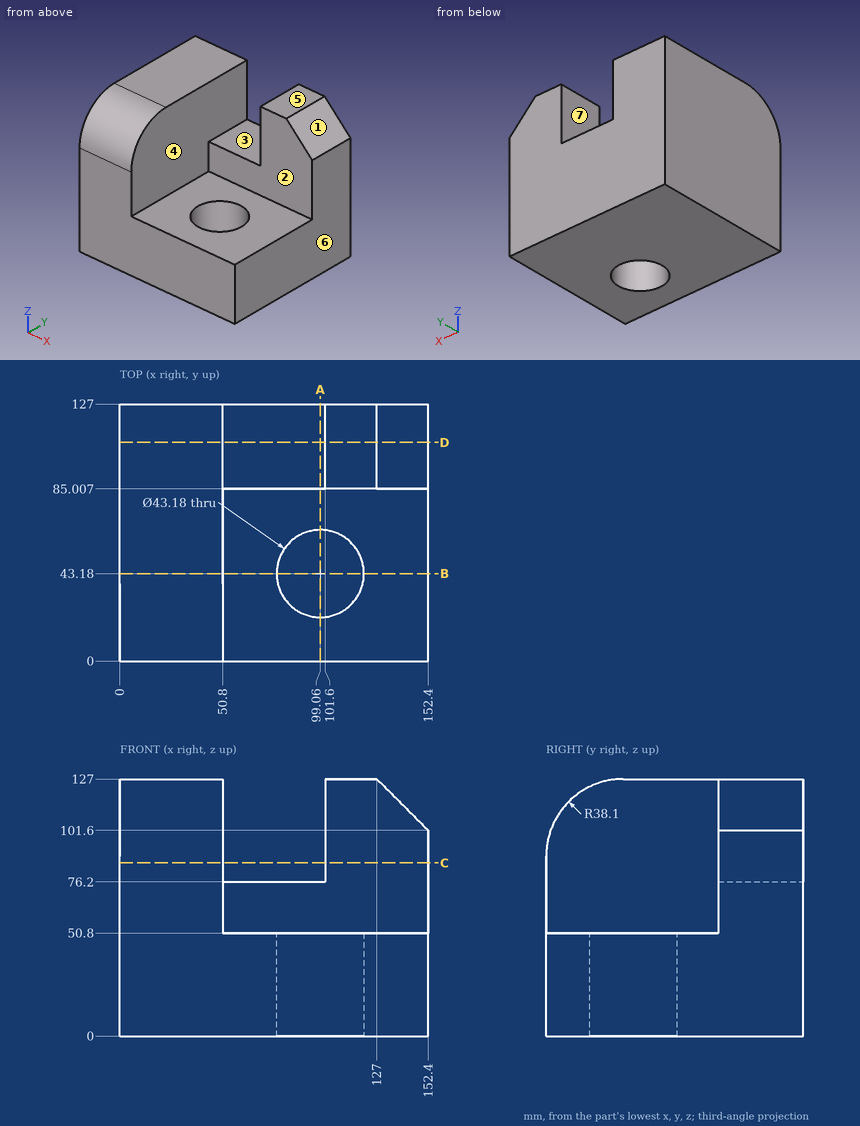
Drawing for the job (mm, zero at the part's lowest x, y, z). A direction names the side the tool comes from. Give positions to 0.01 mm unless a question says otherwise; leave off trailing zeros. Loops run counter-clockwise (first coordinate to the right, second up) from the corner with the lowest first, then second, coordinate; pieces in that order, holes last.
Item 1: Drill centre lines: line 1 along Y through (x, z) = (99.06, 18); line 2 along X through (y, z) = (43, 19); line 3 along Y through (x, z) = (134.5, 109.5). Where is each one in solid material? Low to high.
Check values:
line 1: y = 0 to 21.59, 64.77 to 127
line 2: x = 0 to 77.47, 120.65 to 152.4
line 3: y = 85.01 to 127
Item 2: Slice it at C-C (z = 85.5). Write the cut outline in (x, y).
Check values:
outline: (0, 0) - (50.8, 0) - (50.8, 127) - (0, 127) - close; (101.6, 85.01) - (152.4, 85.01) - (152.4, 127) - (101.6, 127) - close
Item 3: Slice it at D-D (y = 108). Write the cut outline in (x, z).
Check values:
outline: (0, 0) - (152.4, 0) - (152.4, 101.6) - (127, 127) - (101.6, 127) - (101.6, 76.2) - (50.8, 76.2) - (50.8, 127) - (0, 127) - close
Item 4: Which spindle directions (+Z, -Z, +X, -X, +Y, -Y) get a long thin tool onto all of the face, cutting with end or side? Do the marked faces 1, 2, 3 and 4. Say none if no direction does.
Check values:
face 1: +Z, +X, +Y, -Y
face 2: +Z, +X, -Y
face 3: +Z, +Y, -Y
face 4: +Z, -Y
Item 5: Drop flat-ended pins along their axis: P1, Ø8, axis at x = 83, y = 36.5, coming from the +Z side; P2, Ø10, axis at x = 58.5, y = 53, coming from the -Z side; P3, Ø4, axis at y = 68.5, z = 110, coming from the +X side; P4, Ø4, axis at x = 126, y = 64.5, coming from the +Z side. Give the stop position or say it passes through.
Check values:
P1: passes through
P2: stops at z = 0
P3: stops at x = 50.8
P4: stops at z = 50.8
Item 6: Mould opens along X. For the marked faces 5, 6 and 7 say: +X half, -X half, draft (parallel to the pull), parting line (faces both ways), or undercut.
Check values:
face 5: draft
face 6: +X half
face 7: undercut
Item 7: Slice it at B-B (y = 43.18). Write the cut outline in (x, z).
Check values:
outline: (0, 0) - (77.47, 0) - (77.47, 50.8) - (50.8, 50.8) - (50.8, 127) - (0, 127) - close; (120.65, 0) - (152.4, 0) - (152.4, 50.8) - (120.65, 50.8) - close
Item 8: Slice it at A-A (x = 99.06). Write the cut outline in (y, z).
Check values:
outline: (0, 0) - (21.59, 0) - (21.59, 50.8) - (0, 50.8) - close; (64.77, 0) - (127, 0) - (127, 76.2) - (85.01, 76.2) - (85.01, 50.8) - (64.77, 50.8) - close
